Could you check a few things on this model? Use its own coordinates, in mm. A direction names the side the tool comes from. Round coordinates to 2 decimals unless told otherwise and drop trailing zeros. Loops run counter-clockwise (first coordinate to the right, second up) from the corner with the lowest first, then second, coordinate; pieces in that order, holes last. Notation, with made-up numbers: (51.25, 67.25) -> (88.25, 67.25) arc R8 ccw to (88.25, 80.25) -> close; hole circle Ø5 at (12.25, 14.5). An arc over 180 degrees is marked (long way). Put each result on its own line as item: value. Start each with the question number.
1. Which directions (+Z, -Z, +X, -X, +Y, -Y) give clear straight access to the entire face, cutting with the end or side of a thin tool? Please do faces 1 (the flat face through (69, 0, 254)), 2 (the flat face through (71, 51, 0)), 3 (the flat face through (15, 85, -1)).
2. Imagine slicing it at A-A, the plane z = 149. Please give me the cut outline in (x, y).
3. I'm going to push flat-ended pins straight in: P1, Ø3, axis at y = 49, z = 332.5, coming from the -X side; P2, Ø12, axis at x = 106.5, y = 80.5, coming from the +Z side; P3, Ø10, axis at x = 53, z = 309.5, coming from the +Y side. Where does each tip first touch, or does it pass through?
4. Imagine slicing it at B-B, the plane y = 84.5. Please give me the cut outline in (x, z), and give its area (3 significant figures).
5. Imagine slicing it at C-C, the plane x = 14. Please give me the cut outline in (y, z).
6. I need wall thicknesses on line 1 (Y direction, x = 67, z = 113); line 2 (X direction, y = 61.5, z = 400.5). Which ranges of each line are inside material? Lowest first, please. Write a range as [from, to].
```python
from build123d import *

# Parameters (mm, degrees)
TABAN_FLAN_2_DEPTH           = 1.5
KENAR_FLAN_5_STRIP_W         = 7.4732
KENAR_FLAN_5_STRIP_H         = 1.5
KENAR_FLAN_5_STRIP_CUT_DEPTH = 140
KENAR_FLAN_5_DEPTH           = 140
KENAR_FLAN_6_STRIP_W         = 7.4732
KENAR_FLAN_6_STRIP_H         = 1.5
KENAR_FLAN_6_STRIP_CUT_DEPTH = 99.2634
KENAR_FLAN_6_DEPTH           = 99.2634


# Sheet-metal steps are written as plain solids
with BuildPart() as part:
    # Çizim1 → Taban-Flanş2 (new body)
    with BuildSketch(Plane.XY):
        Polygon((0, 0), (0, 70), (30, 100), (140, 100), (140, 0), align=None)
    extrude(amount=-TABAN_FLAN_2_DEPTH)

    # Kenar-Flanş5 strip (across the edge) → Kenar-Flanş5 strip cut (cut)
    with BuildSketch(Plane.YZ):
        with Locations((-3, -0.75)):
            Rectangle(KENAR_FLAN_5_STRIP_W, KENAR_FLAN_5_STRIP_H)
    extrude(amount=KENAR_FLAN_5_STRIP_CUT_DEPTH, mode=Mode.SUBTRACT)

    # Kenar-Flanş5 section (across the edge) → Kenar-Flanş5 (add)
    with BuildSketch(Plane.YZ):
        with BuildLine():
            Line((-1.5, 0.7366), (-1.5, 500))
            Line((-1.5, 500), (0, 500))
            Line((0, 500), (0, 0.7366))
            ThreePointArc((0, 0.7366), (0.215745145, 0.215745145), (0.7366, 0))
            Line((0.7366, 0), (0.7366, -1.5))
            ThreePointArc((0.7366, -1.5), (-0.844915027, -0.844915027), (-1.5, 0.7366))
        make_face()
    extrude(amount=KENAR_FLAN_5_DEPTH)

    # Kenar-Flanş6 strip (across the edge) → Kenar-Flanş6 strip cut (cut)
    with BuildSketch(Plane(origin=(140, 0.7366, 0), x_dir=(-1, 0, 0), z_dir=(0, 1, 0))):
        with Locations((-3, -0.75)):
            Rectangle(KENAR_FLAN_6_STRIP_W, KENAR_FLAN_6_STRIP_H)
    extrude(amount=KENAR_FLAN_6_STRIP_CUT_DEPTH, mode=Mode.SUBTRACT)

    # Kenar-Flanş6 section (across the edge) → Kenar-Flanş6 (add)
    with BuildSketch(Plane(origin=(140, 0.7366, 0), x_dir=(-1, 0, 0), z_dir=(0, 1, 0))):
        with BuildLine():
            Line((-1.5, 0.7366), (-1.5, 500))
            Line((-1.5, 500), (0, 500))
            Line((0, 500), (0, 0.7366))
            ThreePointArc((0, 0.7366), (0.215745145, 0.215745145), (0.7366, 0))
            Line((0.7366, 0), (0.7366, -1.5))
            ThreePointArc((0.7366, -1.5), (-0.844915027, -0.844915027), (-1.5, 0.7366))
        make_face()
    extrude(amount=KENAR_FLAN_6_DEPTH)


solid = part.part
```
Entries:
1. face 1: +Z, +X, -X, +Y
1. face 2: +Z, -X, +Y
1. face 3: +Z, -Z, -X, +Y
2. outline: (0, -1.5) -> (140, -1.5) -> (140, 0) -> (0, 0) -> close; (140, 0.74) -> (141.5, 0.74) -> (141.5, 100) -> (140, 100) -> close
3. P1: x = 140
3. P2: z = 0
3. P3: y = 0
4. outline: (14.5, -1.5) -> (139.26, -1.5) arc R2.24 ccw to (141.5, 0.74) -> (141.5, 500) -> (140, 500) -> (140, 0.74) arc R0.74 cw to (139.26, 0) -> (14.5, 0) -> close
4. area: 940 mm^2
5. outline: (-1.5, 0.74) arc R2.24 ccw to (0.74, -1.5) -> (84, -1.5) -> (84, 0) -> (0.74, 0) arc R0.74 cw to (0, 0.74) -> (0, 500) -> (-1.5, 500) -> close
6. line 1: [-1.5, 0]
6. line 2: [140, 141.5]
